Autodesk Fusion 360 part; units mm, degrees
sketch "Sketch1" plane through (0, 0, 0) normal (0, 0, 1) x (1, 0, 0)
  line L0 (-7.9259, 8.6629) -> (-2.1165, 8.6629)
  line L1 (-1.5, 1) -> (-1.5, -1)
  line L2 (-2.1165, -8.6629) -> (-7.9259, -8.6629)
  line L3 (-7.9259, -8.6629) -> (-7.9259, 8.6629)
  line L4 (2.1165, 8.6629) -> (7.9259, 8.6629)
  line L5 (7.9259, 8.6629) -> (7.9259, -8.6629)
  line L6 (7.9259, -8.6629) -> (2.11, -8.6629)
  line L7 (1.5, -1) -> (1.5, 1)
  line L8 (-48.0743, 0) -> (41.8844, 0) construction
  line L9 (1.5, 18.5935) -> (0, 18.5935) construction
  line L10 (0, 0) -> (0, 17.2446) construction
  line L11 (0, 18.5935) -> (-1.5, 18.5935) construction
  line L12 (-1.5, 1) -> (1.5, 1)
  line L13 (1.5, 1) -> (1.5, -1)
  line L14 (1.5, -1) -> (-1.5, -1)
  line L15 (-1.5, -1) -> (-1.5, 1)
  line L16 (-2.1165, 8.6629) -> (-1.5, 1)
  line L17 (-1.5, -1) -> (-2.1165, -8.6629)
  line L18 (2.11, -8.6629) -> (1.5, -1)
  line L19 (-1.5, -1) -> (-1.5, -18.4253) construction
  line L20 (1.5, 0) -> (7.9259, 0) construction
  line L21 (-1.5, 0) -> (-7.9259, 0) construction
  line L22 (1.5, 1) -> (2.1165, 8.6629)
  line L23 (-1.5, 1) -> (-1.5, 16.5395) construction
  point P0 (1.5, 0)
  point P1 (-1.5, 0)
  point P2 (1.5, 0)
  point P3 (7.9259, 0)
  point P4 (-7.9259, 0)
  dimension "d1" = 4.6
  dimension "d2" = 4.6
  dimension "d3" = 2
  dimension "d8" = 3
extrude "Extrude1" add sketch "Sketch1" along normal blind 14
fillet "Fillet1" radius 1 4 edges at (-1.5, -1, 7) (1.5, -1, 7) (-1.5, 1, 7) (1.5, 1, 7)
equation "d2 = d1"
The listing builds one solid part. Answer for the finished solid, in the listing's coordinates (mm). A direction names the side the tool comes from. Coordinates: 2 decimals unless noted, no trailing zeros. Write each loop counter-clockwise with the first axis right and the second up, starting at its lowest first coordinate (ties: lowest second). Pieces come first, ordered by that corner, then holes. Notation, with made-up numbers: (-20, -24.75) - (-13, -24.75) arc R27 cw to (-13, 12.25) - close; hole circle Ø9 at (10, -23). An arc over 180 degrees is marked (long way). Return JSON: item names as keys, results as strings. Group by question number.
1. Which of the six approach directions +Z, -Z, +X, -X, +Y, -Y give full straight-line access (tool end or side, diameter ignored) to faces 5 (the flat face through (0, 1, 7)), 6 (the flat face through (-7.926, 0, 7)), 7 (the cylindrical face through (1.26, -1.27, 7.1))?
2. A cutting plane is placed at C-C, the plane y = 7. Determine the outline of the cut face in (x, z).
3. A cutting plane is placed at B-B, the plane z = 12. Determine the outline of the cut face in (x, y), plus the area to 3 significant figures.
4. Determine the mould class of faces 1 (the cylindrical face through (-1.25, -1.26, 7.1)), 2 (the flat face through (7.926, 0, 7)), 3 (the flat face through (1.845, -5.339, 6.902)), 4 (the flat face through (-5, -8.663, 7)) for opening direction X: released by +X, released by -X, zero draft, split by the parting line, or undercut.
5. A cutting plane is placed at D-D, the plane x = -1.25. Determine the outline of the cut face in (y, z), plus the area to 3 significant figures.
6. A cutting plane is placed at A-A, the plane y = -4.5. Determine the outline of the cut face in (x, z), plus the area to 3 significant figures.
7. Straight lines are drawn through the part: L1, parallel to X at y = 1.5, z = 1.5; L2, parallel to Y at x = -0.5, z = 9.25; L3, parallel to X at y = 7.25, z = 11. For each, find the intervals that lie inside material, in ascending order.
8. Given pin 1 (0.9 mm diameter, centred on x = 0, z = 10.5, fed in from +Y); pin 2 (0.6 mm diameter, centred on x = -0.5, z = 10, fed in from -Y); pin 3 (6 mm diameter, centred on x = -1.5, y = 5.5, fed in from -Z), each flat-ended and moving along its own axis, determine where each tip first touches the part or whether it passes through.
Ans:
{
 "1": {"face 5": "+Z, -Z, +Y", "face 6": "+Z, -Z, -X, +Y, -Y", "face 7": "+Z, -Z, -Y"},
 "2": {"outline": "(-7.93, 0) - (-1.98, 0) - (-1.98, 14) - (-7.93, 14) - close; (1.98, 0) - (7.93, 0) - (7.93, 14) - (1.98, 14) - close"},
 "3": {"outline": "(-7.93, -8.66) - (-2.12, -8.66) - (-1.57, -1.92) arc R1 cw to (-0.58, -1) - (0.58, -1) arc R1 cw to (1.57, -1.92) - (2.11, -8.66) - (7.93, -8.66) - (7.93, 8.66) - (2.12, 8.66) - (1.57, 1.92) arc R1 cw to (0.58, 1) - (-0.58, 1) arc R1 cw to (-1.57, 1.92) - (-2.12, 8.66) - (-7.93, 8.66) - close", "area": "220 mm²"},
 "4": {"face 1": "undercut", "face 2": "released by +X", "face 3": "undercut", "face 4": "zero draft"},
 "5": {"outline": "(-1.26, 0) - (1.26, 0) - (1.26, 14) - (-1.26, 14) - close", "area": "35.3 mm²"},
 "6": {"outline": "(-7.93, 0) - (-1.78, 0) - (-1.78, 14) - (-7.93, 14) - close; (1.78, 0) - (7.93, 0) - (7.93, 14) - (1.78, 14) - close", "area": "172 mm²"},
 "7": {"L1": "-7.93 to -1.44, 1.44 to 7.93", "L2": "-1 to 1", "L3": "-7.93 to -2, 2 to 7.93"},
 "8": {"pin 1": "y = 1", "pin 2": "y = -1.03", "pin 3": "z = 0"}
}
